Geometry: see drawing. Coordinates: mm, zero at the bounding-box minimum. A direction names the side the tool comes from. Coordinates: 2 decimals unless noted, no trailing zeros. Write each loop counter-clockwise with the first axis right and the second up, starting at its lowest first coordinate (ties: lowest second). Pieces come first, ordered by that corner, then holes.
1) Section query A-A (y = 37). Output: boundary loops of the cut face in (x, z).
2) Set-up query: the marked faces 1, 2 and 3. Return all of +Z, -Z, +X, -X, +Y, -Y with unobstructed straight access to the full face (end or side cutting, diameter ignored); none if empty.
3) Pin query (flat end, axial travel): pin 1 Ø2.5 at (y, z) = (35.5, 38) entering from +X; pin 2 Ø11 at (x, z) = (3, 21) entering from -Y; pin 3 Ø12 at (x, z) = (20.5, 22.5) entering from +Y; pin 4 Ø8 at (x, y) = (15, 47) entering from +Z. Return the tip coordinate at first contact, or that it passes through.
4) Section query C-C (z = 19). Output: boundary loops of the cut face in (x, y), then the cut area to 3 significant figures.
5) Line query: L1, parallel to Y at x = 16, z = 26; L2, parallel to Z at x = 15.5, y = 43; L3, parallel to X at y = 4.5, z = 4.5. Output: solid intervals per line, ascending.
6) Section query D-D (y = 25). Output: boundary loops of the cut face in (x, z), then the cut area to 3 significant figures.
7) Section query B-B (x = 23). Output: boundary loops of the cut face in (y, z).
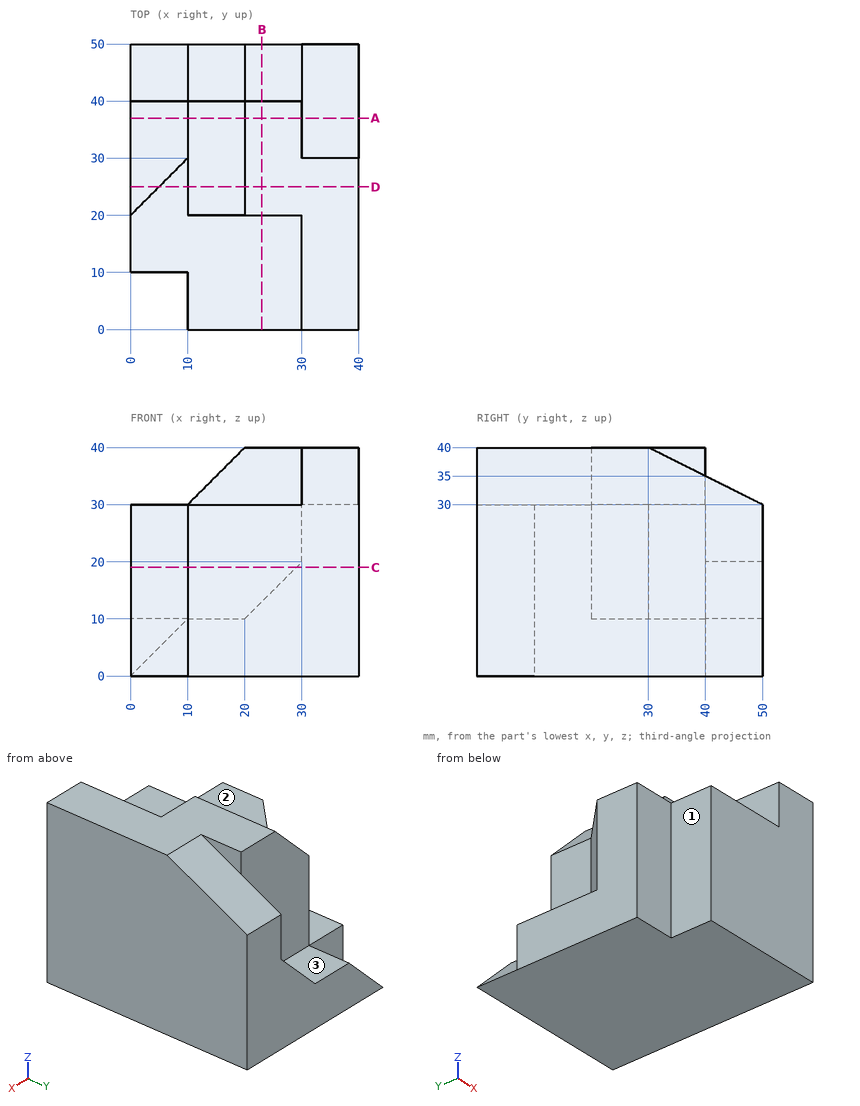
Answer:
1. outline: (0, 0) - (40, 0) - (40, 36.5) - (30, 36.5) - (30, 40) - (20, 40) - (10, 30) - (10, 10) - (0, 10) - close
2. face 1: +Z, -Z, -X, -Y
2. face 2: +Z, -X, -Y
2. face 3: +Z, -X, +Y
3. pin 1: stops at x = 40
3. pin 2: stops at y = 10
3. pin 3: stops at y = 40
3. pin 4: stops at z = 10
4. outline: (0, 10) - (10, 10) - (10, 0) - (40, 0) - (40, 50) - (29, 50) - (29, 40) - (10, 40) - (10, 30) - (0, 20) - close
4. area: 1,460 mm2
5. L1: y = 0 to 40
5. L2: z = 0 to 10
5. L3: x = 10 to 40
6. outline: (0, 0) - (40, 0) - (40, 40) - (20, 40) - (10, 30) - (5, 30) - (5, 10) - (0, 10) - close
6. area: 1,350 mm2
7. outline: (0, 0) - (50, 0) - (50, 13) - (40, 13) - (40, 40) - (20, 40) - (20, 30) - (0, 30) - close
